Geometry: final body of the model. Coordinates: model frame, mm. A direction names the side the tool comes from. Give positions to 0.01 mm unless a question says otherwise; leave off trailing zeros. Write each loop counter-clockwise with the first axis right and the second up, starting at its lowest first coordinate (ties: lowest second). Pieces come first, ordered by that corner, then holes. Notation, with made-up numbers: M 31.25,67 L 90.25,67 A7 cw 90.25,77 Z; hole C 15,54 d3. An arc over 180 degrees is marked long. Use one line per item in the form item = value. Start each with the question number.
Item 1: Contact query for flat-ended pins moving along their axis: P1, Ø6, axis at y = -25.5, z = 40.5, coming from the +X side; P2, Ø20, axis at y = -33, z = 46, coming from the +X side; P3, Ø12, axis at x = 75.5, y = -16, coming from the +Z side. Output: stop coordinate, or through.
Item 2: Section query C-C on x = 168. Return loops of the section in (y, z), then the cut area to 3 significant figures.
Item 3: Material intervals for line 1 along X through (y, z) = (-42, 50.5); line 2 along Z through (x, y) = (184, -41.5); line 3 along Z through (x, y) = (64.5, -51), sorted ascending. Write a range as from..to.
Item 4: Section query D-D on z = 35. Return loops of the section in (x, y).
Item 5: Section query A-A on z = 56. Return loops of the section in (x, y).
Item 6: Section query B-B on y = -20. Return loops of the section in (x, z).
Item 7: Pull-direction query (X, two-part tool) for faces 3 (the flat face through (200, -30, 23)), 4 (the flat face through (140, -30, 54)), 5 (the flat face through (0, -30, 30)), 6 (the flat face through (60, -30, 40)); classes: released by +X, released by -X, zero draft, split by the parting line, or undercut.
Item 8: Access query for faces 1 (the flat face through (99, -30, 0)), 2 (the flat face through (101, -30, 20)). Directions: +Z, -Z, +X, -X, +Y, -Y. A direction counts if a zero-diameter tool reaches every point of the face in a straight line with its end or side. Return the directions, or none.
from build123d import *

# Parameters (mm, degrees)
F1_DEPTH = 60
F3_DEPTH = 60
F4_R     = 10


with BuildPart() as f1:
    # F0 (on Front) → F1 (new body)
    with BuildSketch(Plane.XZ):
        Polygon((0, 60), (0, 0), (200, 0), (200, 60), (140, 60), (140, 20), (60, 20), (60, 60), align=None)
    extrude(amount=F1_DEPTH)

    # F2 (on face) → F3 (cut)
    with BuildSketch(Plane.YZ.offset(200)):
        with BuildLine():
            Line((-30, 40), (-17.5, 40))
            ThreePointArc((-17.5, 40), (-21.1611652352, 48.8388347648), (-30, 52.5))
            Line((-30, 52.5), (-30, 40))
        make_face()
        with BuildLine():
            Line((-30, 40), (-30, 52.5))
            ThreePointArc((-30, 52.5), (-38.8388347648, 48.8388347648), (-42.5, 40))
            Line((-42.5, 40), (-30, 40))
        make_face()
        with BuildLine():
            ThreePointArc((-42.5, 40), (-38.8388347648, 31.1611652352), (-30, 27.5))
            Line((-30, 27.5), (-30, 40))
            Line((-30, 40), (-42.5, 40))
        make_face()
        with BuildLine():
            ThreePointArc((-30, 27.5), (-21.1611652352, 31.1611652352), (-17.5, 40))
            Line((-17.5, 40), (-30, 40))
            Line((-30, 40), (-30, 27.5))
        make_face()
    extrude(amount=-F3_DEPTH, mode=Mode.SUBTRACT)

    # F4
    f4_edges = [f1.edges().sort_by_distance(p)[0] for p in [
        (0, 0, 30),
        (0, -60, 30),
    ]]
    fillet(f4_edges, radius=F4_R)


solid = f1.part
Answer sheet:
q1.P1 = 60
q1.P2 = 200
q1.P3 = 20
q2.outline = M -60,0 L 0,0 L 0,60 L -60,60 Z; hole C -30,40 d25
q2.area = 3,110 mm2
q3.line_1 = 0..60, 140..200
q3.line_2 = 0..35.1, 44.9..60
q3.line_3 = 0..20
q4.outline = M 0,-50 A10 ccw 10,-60 L 60,-60 L 60,0 L 10,0 A10 ccw 0,-10 Z; M 140,-60 L 200,-60 L 200,-41.46 L 140,-41.46 Z; M 140,-18.54 L 200,-18.54 L 200,0 L 140,0 Z
q5.outline = M 0,-50 A10 ccw 10,-60 L 60,-60 L 60,0 L 10,0 A10 ccw 0,-10 Z; M 140,-60 L 200,-60 L 200,0 L 140,0 Z
q6.outline = M 0,0 L 200,0 L 200,32.5 L 140,32.5 L 140,20 L 60,20 L 60,60 L 0,60 Z; M 140,47.5 L 200,47.5 L 200,60 L 140,60 Z
q7.face_3 = released by +X
q7.face_4 = undercut
q7.face_5 = released by -X
q7.face_6 = undercut
q8.face_1 = -Z, +X, -X, +Y, -Y
q8.face_2 = +Z, +Y, -Y
